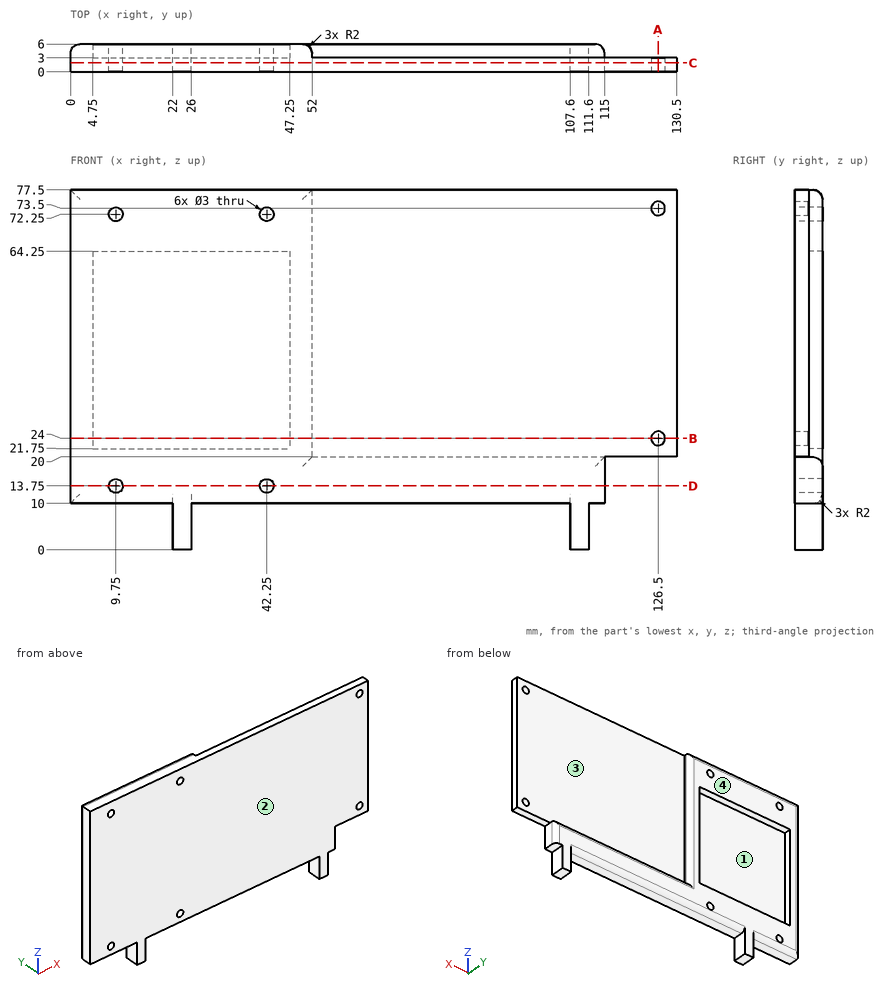
Geometry: see drawing. Coordinates: mm, zero at the bounding-box minimum. A direction names the side the tool comes from. Round coordinates to 2 decimals unless told otherwise and drop trailing zeros. Write each loop counter-clockwise with the first axis right and the second up, starting at its lowest first coordinate (ties: lowest second). Pieces come first, ordered by that corner, then holes.
1) Cut plane A-A (x = 126.5). Return the cut outline in (y, z), then the cut area to 4 significant figures.
2) Contact query for flat-ended pins moving along their axis: P1, Ø2.5, axis at x = 9.75, z = 72.25, coming from the +Y side; P2, Ø3, axis at y = 1.5, z = 8, coming from the -X side; P3, Ø5, axis at x = 97, z = 31.5, coming from the +Y side; P4, Ø2, axis at x = 105, y = 4.5, coming from the -Z side. Output: stop coordinate, or through.
3) Reachability of the marked faces 3 and 4 from +Z, -Z, +X, -X, +Y, -Y: full face, straight path, thin tool, end or side. Return the list, or none.
4) Cut plane C-C (y = 1.95). Return the cut outline in (x, z).
5) Ray query, L1, parallel to X at y = 2.9, z = 13.75; L2, parallel to Z at x = 126.5, y = 0.9; L3, parallel to Z at x = 43, y = 5.4. Return the intervals inside material, ascending.
6) Draft query along Z for the marked faces 1 and 2. Return one class per face: pulls with the +Z half, pulls with the -Z half, needs draft (parallel to the pull), parting line crosses it, or undercut.
7) Cut plane D-D (z = 13.75). Return the cut outline in (x, y).
8) Cut plane B-B (z = 24). Return the cut outline in (x, y).
Geometry says:
1. outline: (0, 20) - (3, 20) - (3, 22.5) - (0, 22.5) - close; (0, 25.5) - (3, 25.5) - (3, 72) - (0, 72) - close; (0, 75) - (3, 75) - (3, 77.5) - (0, 77.5) - close
1. area: 154.5 mm2
2. P1: passes through
2. P2: stops at x = 22
2. P3: stops at y = 3
2. P4: stops at z = 10
3. face 3: +Z, +X, +Y
3. face 4: +Z, -Z, +X, -X, +Y
4. outline: (0, 10) - (22, 10) - (22, 0) - (26, 0) - (26, 10) - (107.6, 10) - (107.6, 0) - (111.6, 0) - (111.6, 10) - (115, 10) - (115, 20) - (130.5, 20) - (130.5, 77.5) - (0, 77.5) - close; hole circle Ø3 at (9.75, 13.75); hole circle Ø3 at (9.75, 72.25); hole circle Ø3 at (42.25, 13.75); hole circle Ø3 at (42.25, 72.25); hole circle Ø3 at (126.5, 24); hole circle Ø3 at (126.5, 73.5)
5. L1: x = 0 to 8.25, 11.25 to 40.75, 43.75 to 115
5. L2: z = 20 to 22.5, 25.5 to 72, 75 to 77.5
5. L3: z = 10.57 to 12.45, 15.05 to 21.75, 64.25 to 70.95, 73.55 to 76.93
6. face 1: undercut
6. face 2: needs draft
7. outline: (0, 0) - (8.25, 0) - (8.25, 6) - (2, 6) arc R2 ccw to (0, 4) - close; (11.25, 0) - (40.75, 0) - (40.75, 6) - (11.25, 6) - close; (43.75, 0) - (115, 0) - (115, 4) arc R2 ccw to (113, 6) - (43.75, 6) - close
8. outline: (0, 0) - (125, 0) - (125, 3) - (52, 3) - (52, 4) arc R2 ccw to (50, 6) - (47.25, 6) - (47.25, 3) - (4.75, 3) - (4.75, 6) - (2, 6) arc R2 ccw to (0, 4) - close; (128, 0) - (130.5, 0) - (130.5, 3) - (128, 3) - close
